CAD build for the part. Positions are in the model's coordinates, mm. Coordinates: 2 decimals unless noted, no trailing zeros. Write each loop counter-clockwise with the first axis right and the second up, starting at its lowest first coordinate (ties: lowest second). Pieces come first, ordered by that corner, then holes.
Autodesk Inventor part; units mm, degrees
ref_plane "YZ Plane" through (0, 0, 0) normal (1, 0, 0) x (0, 1, 0)
ref_plane "XZ Plane" through (0, 0, 0) normal (0, 1, 0) x (-1, 0, 0)
ref_plane "XY Plane" through (0, 0, 0) normal (0, 0, 1) x (1, 0, 0)
sketch "Sketch1" plane through (0, 0, 0) normal (0, 0, 1) x (1, 0, 0)
  line L0 (-57.7612, 63.8108) -> (18.4388, 63.8108)
  line L1 (18.4388, 63.8108) -> (18.4388, -22.1174)
  line L2 (18.4388, -22.1174) -> (-57.7612, -22.1174)
  line L3 (-57.7612, -22.1174) -> (-57.7612, 63.8108)
  line L4 (-57.7612, 63.8108) -> (-48.2362, 63.8108)
  line L5 (-48.2362, 63.8108) -> (-48.2362, 54.2858)
  line L6 (18.4388, 63.8108) -> (8.9138, 63.8108)
  line L7 (8.9138, 63.8108) -> (8.9138, 54.2858)
  line L8 (-57.7612, -22.1174) -> (-57.7612, -12.5924)
  line L9 (-57.7612, -12.5924) -> (-48.2362, -12.5924)
  circle A0 centre (-48.2362, 54.2858) radius 2.0193
  circle A1 centre (8.9138, 54.2858) radius 2.0193
  circle A2 centre (-48.2362, -12.5924) radius 2.0193
  circle A3 centre (8.9138, -12.5924) radius 2.0193
  circle A4 centre (-51.7612, 20.8467) radius 3.048
  circle A5 centre (12.4388, 20.8467) radius 3.048
  point P0 (0, 0)
  dimension "d0" = 76.2
  dimension "d1" = 85.9282
  dimension "d2" = 9.525
  dimension "d3" = 9.525
  dimension "d4" = 9.525
  dimension "d5" = 9.525
  dimension "d6" = 9.525
  dimension "d7" = 9.525
  dimension "d8" = 4.0386
  dimension "d9" = 4.0386
  dimension "d10" = 4.0386
  dimension "d11" = 4.0386
  dimension "d15" = 6.096
  dimension "d16" = 6.096
extrude "Extrusion1" add sketch "Sketch1" along normal blind 6.35
sketch "Sketch2" plane through (0, 0, 6.35) normal (0, 0, 1) x (1, 0, 0)
  circle A0 centre (12.4388, 20.8467) radius 3.048
  circle A1 centre (-51.7612, 20.8467) radius 3.048
  circle A2 centre (-51.7612, 20.8467) radius 3.048
  circle A3 centre (12.4388, 20.8467) radius 3.048
  point P0 (0, 0)
hole "Hole1" at (-51.7612, 20.8467, 6.35) at (12.4388, 20.8467, 6.35) direction (0, 0, -1) diameter 6.35 depth 25.4 tip angle 118 countersink diameter 9.525 countersink angle 82
properties part number "glass socket bottom"
Item 1: Two-plate mould, pull along X, no slides. Class faces 1 (the flat face through (-19, -22.117, 3)), 2 (the cylindrical face through (-48.66, 21.53, 2.23)), 3 (the flat face through (18.439, 21, 3)): +X half, -X half, draft (parallel to the pull), parting line (faces both ways), or undercut.
Item 2: Saw through at A-A, the plane z = 2. Write the cut outline in (x, y) (3 decimals), and give its area (3 significant figures).
Item 3: Wall check: line 1 along Y through (x, z) = (9, 1.5); line 2 along X through (y, z) = (54, 3.25); line 3 along Y through (x, z) = (-50, 3.25). Give the ranges that are in metal, low to high.
Working result:
1. face 1: draft
1. face 2: undercut
1. face 3: +X half
2. outline: (-57.761, -22.117) - (18.439, -22.117) - (18.439, 63.811) - (-57.761, 63.811) - close; hole circle Ø6.35 at (-51.761, 20.847); hole circle Ø4.039 at (-48.236, -12.592); hole circle Ø4.039 at (-48.236, 54.286); hole circle Ø4.039 at (8.914, -12.592); hole circle Ø4.039 at (8.914, 54.286); hole circle Ø6.35 at (12.439, 20.847)
2. area: 6,430 mm2
3. line 1: y = -22.12 to -14.61, -10.57 to 52.27, 56.3 to 63.81
3. line 2: x = -57.76 to -50.24, -46.24 to 6.91, 10.91 to 18.44
3. line 3: y = -22.12 to -13.58, -11.61 to 18.2, 23.49 to 53.3, 55.27 to 63.81
